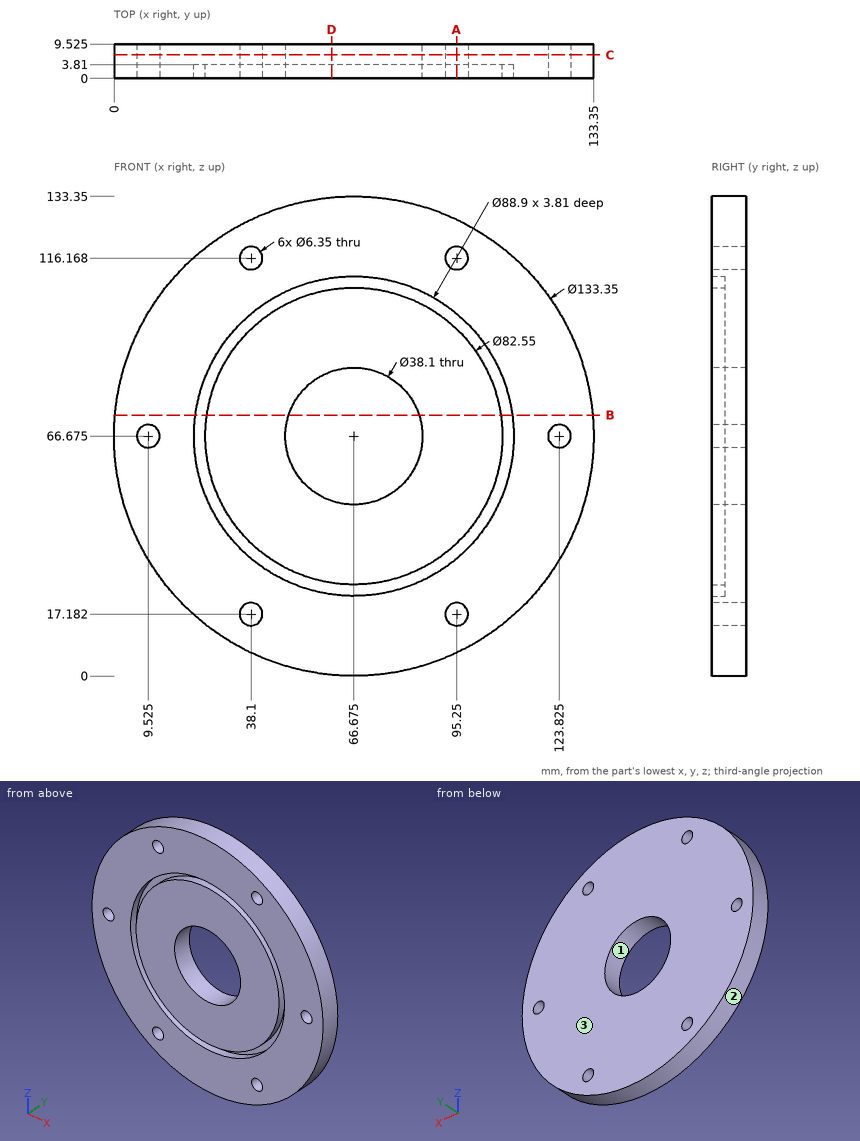
Check sheet for the drawn part. Datum: minimum x, y, z corner. Units: mm. Coordinates: 2 decimals unless noted, no trailing zeros. Loops run counter-clockwise (first coordinate to the right, second up) from the corner with the lowest first, then second, coordinate; pieces in that order, holes last. Notation, with made-up numbers: (6.25, 23) -> (25.25, 23) arc R35 cw to (25.25, 62) -> close; hole circle Ø9 at (-4, 76.5). An arc over 180 degrees is marked (long way). Answer as CSV lines item,"result".
1) Thickness scan on L1, parallel to X at y = 3.75, z = 113.5; L2, parallel to X at y = 3.25, z = 40; L3, parallel to X at y = 3.25, z = 70.5. Record the ranges inside material, lowest first. Write a range as from..to.
Found:
L1,"x = 19.21..36.38, 39.82..93.53, 96.97..114.14"
L2,"x = 5.57..31.12, 35.18..98.17, 102.23..127.78"
L3,"x = 0.11..22.39, 25.58..48.01, 85.34..107.77, 110.96..133.24"
2) Cross-section at D-D, the plane x = 60.5. Record the cut outline in (y, z) (1 decimal).
Found:
outline,"(0, 0.3) -> (9.5, 0.3) -> (9.5, 48.7) -> (0, 48.7) -> (0, 25.9) -> (3.8, 25.9) -> (3.8, 22.7) -> (0, 22.7) -> close; (0, 84.7) -> (9.5, 84.7) -> (9.5, 133.1) -> (0, 133.1) -> (0, 110.7) -> (3.8, 110.7) -> (3.8, 107.5) -> (0, 107.5) -> close"
3) Cross-section at C-C, the plane y = 6.5. Count the separate pieces of the cut face and the enclosed holes in it, then the cut area to 3 significant figures.
Found:
separate pieces,"1"
enclosed holes,"7"
area,"12,600 mm2"
4) Depth check by flat-ended pin: pin 1 (10 mm diameter, centred on x = 38.1, z = 17.18, fed in from -Y); pin 2 (5.5 mm diameter, centred on x = 123.825, z = 66.675, fed in from +Y); pin 3 (2 mm diameter, centred on y = 6.5, z = 118.5, fed in from +X); pin 4 (5 mm diameter, centred on x = 74.5, y = 8.5, fed in from -Z). Enter the tip coordinate at first touch or a pass-through.
Found:
pin 1,"stops at y = 0"
pin 2,"passes through"
pin 3,"stops at x = 109.83"
pin 4,"stops at z = 0.21"
5) Cross-section at B-B, the plane z = 72.5. Record the cut outline in (x, y) (1 decimal).
Found:
outline,"(0.3, 0) -> (22.6, 0) -> (22.6, 3.8) -> (25.8, 3.8) -> (25.8, 0) -> (48.5, 0) -> (48.5, 9.5) -> (0.3, 9.5) -> close; (84.8, 0) -> (107.5, 0) -> (107.5, 3.8) -> (110.7, 3.8) -> (110.7, 0) -> (133.1, 0) -> (133.1, 9.5) -> (84.8, 9.5) -> close"
6) Release check for a two-part mould opening along X. For the marked faces 1, 2 and 3 record: +X half, -X half, draft (parallel to the pull), parting line (faces both ways), or undercut.
Found:
face 1,"undercut"
face 2,"parting line"
face 3,"draft"
7) Cross-section at A-A, the plane x = 95.25. Record the cut outline in (y, z) (1 decimal), then the cut area to 3 significant figures.
Found:
outline,"(0, 6.4) -> (9.5, 6.4) -> (9.5, 14) -> (0, 14) -> close; (0, 20.4) -> (9.5, 20.4) -> (9.5, 113) -> (0, 113) -> (0, 100.7) -> (3.8, 100.7) -> (3.8, 96.5) -> (0, 96.5) -> (0, 36.9) -> (3.8, 36.9) -> (3.8, 32.6) -> (0, 32.6) -> close; (0, 119.3) -> (9.5, 119.3) -> (9.5, 126.9) -> (0, 126.9) -> close"
area,"994 mm2"
